```python
from build123d import *

# Parameters (mm, degrees)
F0_R     = 15.5998218224
F1_DEPTH = 25.4


# Not quite as in the source:
# - a feature of the source that left no trace in its solid (it failed there, or was rolled back) is left out


with BuildPart() as f1:
    # F0 (on Top) → F1 (new body)
    with BuildSketch(Plane.XY):
        with BuildLine():
            Line((-9.7679234278, 31.6427110991), (-12.2910759721, 33.8783473239))
            Line((-12.2910759721, 33.8783473239), (-9.6983198699, 46.5739309325))
            Line((-9.6983198699, 46.5739309325), (2.5927561023, 50.6763300865))
            Line((2.5927561023, 50.6763300865), (12.2910759721, 42.0831456318))
            Line((12.2910759721, 42.0831456318), (9.6983198699, 29.3875620231))
            Line((9.6983198699, 29.3875620231), (8.1033290175, 28.8552010534))
            ThreePointArc((8.1033290175, 28.8552010534), (8.7164308394, 26.6457057993), (9.4057371171, 24.4587855955))
            ThreePointArc((9.4057371171, 24.4587855955), (14.5985992918, 30.3523642419), (16.4715304941, 37.9807464778))
            ThreePointArc((16.4715304941, 37.9807464778), (-6.8274979981, 52.9706293294), (-10.8114943571, 25.5540451221))
            ThreePointArc((-10.8114943571, 25.5540451221), (-10.2185999519, 28.5861903467), (-9.7679234278, 31.6427110991))
        make_face()
        with BuildLine():
            Line((-2.5927561023, 25.2851628692), (-9.7679234278, 31.6427110991))
            ThreePointArc((-9.7679234278, 31.6427110991), (-10.2185999519, 28.5861903467), (-10.8114943571, 25.5540451221))
            ThreePointArc((-10.8114943571, 25.5540451221), (-0.8910312632, 21.5333339121), (9.4057371171, 24.4587855955))
            ThreePointArc((9.4057371171, 24.4587855955), (8.7164308394, 26.6457057993), (8.1033290175, 28.8552010534))
            Line((8.1033290175, 28.8552010534), (-2.5927561023, 25.2851628692))
        make_face()
        with BuildLine():
            ThreePointArc((9.4057371171, 24.4587855955), (-0.8910312632, 21.5333339121), (-10.8114943571, 25.5540451221))
            ThreePointArc((-10.8114943571, 25.5540451221), (-16.4556801257, 9.772653233), (-25.88479823, -4.083785513))
            ThreePointArc((-25.88479823, -4.083785513), (-27.4340735437, -5.7742023624), (-29.0410016523, -7.4099117424))
            Line((-29.0410016523, -7.4099117424), (-20.6012153324, -14.887974085))
            Line((-20.6012153324, -14.887974085), (-22.5194299425, -24.2806253802))
            ThreePointArc((-22.5194299425, -24.2806253802), (-19.6470670617, -23.1426623228), (-16.7247050666, -22.1400513271))
            ThreePointArc((-16.7247050666, -22.1400513271), (-0.2355258993, -19.1373636419), (16.4790611129, -20.3750000825))
            ThreePointArc((16.4790611129, -20.3750000825), (19.0939298277, -9.9950112466), (27.5361994237, -3.4139937949))
            ThreePointArc((27.5361994237, -3.4139937949), (16.691206025, 9.3647104089), (9.4057371171, 24.4587855955))
        make_face()
        Circle(F0_R, mode=Mode.SUBTRACT)
        with BuildLine():
            ThreePointArc((-29.0410016523, -7.4099117424), (-27.4340735437, -5.7742023624), (-25.88479823, -4.083785513))
            ThreePointArc((-25.88479823, -4.083785513), (-47.5816840445, -26.4424238123), (-16.7247050666, -22.1400513271))
            ThreePointArc((-16.7247050666, -22.1400513271), (-19.6470670617, -23.1426623228), (-22.5194299425, -24.2806253802))
            Line((-22.5194299425, -24.2806253802), (-23.1939714347, -27.5835576936))
            Line((-23.1939714347, -27.5835576936), (-35.4850474068, -31.6859568476))
            Line((-35.4850474068, -31.6859568476), (-45.1833672766, -23.0927723929))
            Line((-45.1833672766, -23.0927723929), (-42.5906111744, -10.3971887842))
            Line((-42.5906111744, -10.3971887842), (-30.2995352023, -6.2947896303))
            Line((-30.2995352023, -6.2947896303), (-29.0410016523, -7.4099117424))
        make_face()
        with BuildLine():
            ThreePointArc((49.3638217986, -18.9903732389), (42.4601616546, -5.5826451025), (27.5361994237, -3.4139937949))
            ThreePointArc((27.5361994237, -3.4139937949), (29.8656670136, -5.4435280239), (32.2873533703, -7.3620857189))
            Line((32.2873533703, -7.3620857189), (35.4850474068, -6.2947896303))
            Line((35.4850474068, -6.2947896303), (45.1833672766, -14.887974085))
            Line((45.1833672766, -14.887974085), (42.5906111744, -27.5835576936))
            Line((42.5906111744, -27.5835576936), (30.2995352023, -31.6859568476))
            Line((30.2995352023, -31.6859568476), (20.6012153324, -23.0927723929))
            Line((20.6012153324, -23.0927723929), (20.9376726348, -21.4452893111))
            ThreePointArc((20.9376726348, -21.4452893111), (18.7176427043, -20.8715034369), (16.4790611129, -20.3750000825))
            ThreePointArc((16.4790611129, -20.3750000825), (33.5852181443, -35.4473222032), (49.3638217986, -18.9903732389))
        make_face()
        with BuildLine():
            ThreePointArc((32.2873533703, -7.3620857189), (29.8656670136, -5.4435280239), (27.5361994237, -3.4139937949))
            ThreePointArc((27.5361994237, -3.4139937949), (19.0939298277, -9.9950112466), (16.4790611129, -20.3750000825))
            ThreePointArc((16.4790611129, -20.3750000825), (18.7176427043, -20.8715034369), (20.9376726348, -21.4452893111))
            Line((20.9376726348, -21.4452893111), (23.1939714347, -10.3971887842))
            Line((23.1939714347, -10.3971887842), (32.2873533703, -7.3620857189))
        make_face()
    extrude(amount=F1_DEPTH)


solid = f1.part
```
The listing builds one solid part. Answer for the finished solid, in the listing's coordinates (mm). A direction names the side the tool comes from. Coordinates: 2 decimals unless noted, no trailing zeros. Loops run counter-clockwise (first coordinate to the right, second up) from the corner with the lowest first, then second, coordinate; pieces in that order, holes last. Notation, with made-up numbers: (-10, 60) -> (48, 60) arc R26 cw to (48, 94) -> close; hole circle Ø2 at (88, 29). An arc over 180 degrees is marked (long way). Use one line per item in the form item = value. Start each with the question number.
Item 1: Consider L1, parallel to Y at x = 0, z = 17.25; L2, parallel to X at y = -27, z = 13.5; L3, parallel to X at y = -17.5, z = 11.5. Determine where each line is inside the solid, lowest interval first. Write a range as [from, to].
Item 2: A tool of negligible diameter and unlimited length cuts with its end or side. For faces 1 (the face through (-0.47, -19.15, 12.52)), 2 (the face through (-40.266, -27.45, 12.522)), from which of +Z, -Z, +X, -X, +Y, -Y can it reach the whole face along a straight path? Write none if from no direction.
Item 3: The part is cut by section C-C on x = 0. Determine the outline of the cut face in (y, z), then the cut area to 3 significant figures.
Item 4: The part is cut by section B-B on z = 11.25. Determine the outline of the cut face in (x, y) (1 decimal), then the cut area to 3 significant figures.
Item 5: The mould has two halves that part along X. Classify faces 3 (the face through (-47.83, -25.93, 12.52)), 4 (the face through (-29.253, -29.606, 12.522)), 5 (the face through (0, -17, 0)): released by +X, released by -X, zero draft, split by the parting line, or undercut.
Item 6: The part is cut by section A-A on y = 0. Determine the outline of the cut face in (x, z), then the cut area to 3 significant figures.
Item 7: The part is cut by section D-D on y = 12. Determine the outline of the cut face in (x, z).
Item 8: Flat-ended cylindrical pins translate along their axes: pin 1 Ø8 at (x, z) = (-7.5, 19) entering from -Y; pin 2 Ø2 at (y, z) = (-1, 13.5) entering from +X; pin 3 Ø2 at (y, z) = (-15.5, 3) entering from -X. Find the tip coordinate at first contact, or state that the pin passes through.
Answer key:
q1.L1 = [-19.13, -15.6], [15.6, 26.15], [49.81, 54.45]
q1.L2 = [-47.29, -40.77], [-23.07, -18.5], [18.5, 25.01], [42.71, 47.29]
q1.L3 = [-49.3, -44.04], [-21.13, 21.74], [44.65, 49.3]
q2.face_1 = +Z, -Z, -Y
q2.face_2 = +Z, -Z
q3.outline = (-19.13, 0) -> (-15.6, 0) -> (-15.6, 25.4) -> (-19.13, 25.4) -> close; (15.6, 0) -> (26.15, 0) -> (26.15, 25.4) -> (15.6, 25.4) -> close; (49.81, 0) -> (54.45, 0) -> (54.45, 25.4) -> (49.81, 25.4) -> close
q3.area = 475 mm2
q4.outline = (-25.9, -4.1) arc R16.5 ccw (long way) to (-16.7, -22.1) arc R66.2 cw to (16.5, -20.4) arc R16.5 ccw (long way) to (27.5, -3.4) arc R66.2 cw to (9.4, 24.5) arc R16.5 ccw (long way) to (-10.8, 25.6) arc R66.2 cw to start; hole (-45.2, -23.1) -> (-35.5, -31.7) -> (-23.2, -27.6) -> (-20.6, -14.9) -> (-30.3, -6.3) -> (-42.6, -10.4) -> close; hole circle Ø31.2 at (0, 0); hole (-12.3, 33.9) -> (-2.6, 25.3) -> (9.7, 29.4) -> (12.3, 42.1) -> (2.6, 50.7) -> (-9.7, 46.6) -> close; hole (20.6, -23.1) -> (30.3, -31.7) -> (42.6, -27.6) -> (45.2, -14.9) -> (35.5, -6.3) -> (23.2, -10.4) -> close
q4.area = 2,010 mm2
q5.face_3 = undercut
q5.face_4 = undercut
q5.face_5 = zero draft
q6.outline = (-22.55, 0) -> (-15.6, 0) -> (-15.6, 25.4) -> (-22.55, 25.4) -> close; (15.6, 0) -> (24.06, 0) -> (24.06, 25.4) -> (15.6, 25.4) -> close
q6.area = 392 mm2
q7.outline = (-15.37, 0) -> (-9.97, 0) -> (-9.97, 25.4) -> (-15.37, 25.4) -> close; (9.97, 0) -> (15.06, 0) -> (15.06, 25.4) -> (9.97, 25.4) -> close
q8.pin_1 = -20.72
q8.pin_2 = 26.04
q8.pin_3 = -49.17
